from build123d import *

# Parameters (mm, degrees)
SKETCH1_W           = 5
SKETCH1_H           = 159
BOSS_EXTRUDE1_DEPTH = 3
SKETCH3_W           = 23
SKETCH3_H           = 5
BOSS_EXTRUDE2_DEPTH = 3
SKETCH5_R           = 1
CUT_EXTRUDE4_DEPTH  = 3


with BuildPart() as part:
    # Sketch1 → Boss-Extrude1 (new body)
    with BuildSketch(Plane(origin=(0, 0, 0), x_dir=(1, 0, 0), z_dir=(0, 1, 0))):
        with Locations((2.5, 79.5)):
            Rectangle(SKETCH1_W, SKETCH1_H)
    extrude(amount=BOSS_EXTRUDE1_DEPTH)

    # Sketch3 → Boss-Extrude2 (add)
    with BuildSketch(Plane(origin=(0, 0, 0), x_dir=(1, 0, 0), z_dir=(0, 1, 0))):
        with Locations((2.5, 12.5)):
            Rectangle(SKETCH3_W, SKETCH3_H)
        with Locations((2.5, 146.5)):
            Rectangle(SKETCH3_W, SKETCH3_H)
    extrude(amount=BOSS_EXTRUDE2_DEPTH)

    # Sketch5 → Cut-Extrude4 (cut)
    with BuildSketch(Plane(origin=(0, 0, 0), x_dir=(1, 0, 0), z_dir=(0, 1, 0))):
        with Locations((2.5, 12.5)):
            Circle(SKETCH5_R)
        with Locations((2.5, 146.5)):
            Circle(SKETCH5_R)
    extrude(amount=CUT_EXTRUDE4_DEPTH, mode=Mode.SUBTRACT)


solid = part.part
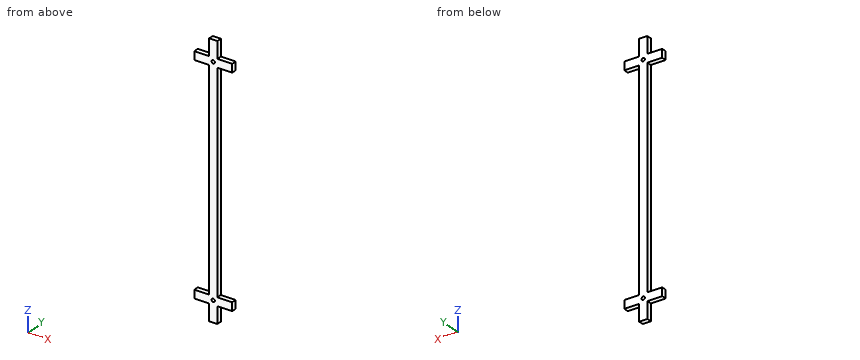
Can you work these out from the model? Positions are in its coordinate system, mm. Round coordinates to 2 decimals unless told otherwise and drop trailing zeros. Loops run counter-clockwise (first coordinate to the right, second up) from the corner with the lowest first, then second, coordinate; pieces in that order, holes last. Notation, with made-up numbers: (7, 2) - (49, 2) arc R15 cw to (49, 7) - close; hole circle Ø3 at (43.25, 2.25). An arc over 180 degrees is marked (long way). Write item = value, one per line. Start each with the question number.
(1) If we section it at A-A (y = 0.7): Please give me the cut outline in (x, z), and give its area (3 significant figures).
(2) If we section it at B-B (x = -2.75): Please give me the cut outline in (y, z), and give its area (3 significant figures).
(3) If we section it at C-C (z = -120.5): Please give me the cut outline in (x, y), and give its area (3 significant figures).
(4) If I drill on probe 1 along Z at (x, y) = (2.5, 1.5); probe 2 along Z at (x, y) = (-2.5, 0.9); probe 3 along X at (y, z) = (2.3, -146.5), over which ranges is the centre line in solid material (lowest first)? Write a range as [from, to].
(5) For P1, Ø0.9, axis at x = -2.5, y = 1, coming from the -Z side; P2, Ø1, axis at x = -2.5, y = 1.5, coming from the +Z side; P3, Ø1.5, axis at y = 1.5, z = -48, coming from the -X side, each with a flat end and sliding along its axis, tell me the tip position at first contact or that it passes through.
Ans:
q1.outline = (-9, -149) - (0, -149) - (0, -159) - (5, -159) - (5, -149) - (14, -149) - (14, -144) - (5, -144) - (5, -15) - (14, -15) - (14, -10) - (5, -10) - (5, 0) - (0, 0) - (0, -10) - (-9, -10) - (-9, -15) - (0, -15) - (0, -144) - (-9, -144) - close; hole circle Ø2 at (2.5, -146.5); hole circle Ø2 at (2.5, -12.5)
q1.area = 969 mm²
q2.outline = (0, -149) - (3, -149) - (3, -144) - (0, -144) - close; (0, -15) - (3, -15) - (3, -10) - (0, -10) - close
q2.area = 30.0 mm²
q3.outline = (0, 0) - (5, 0) - (5, 3) - (0, 3) - close
q3.area = 15.0 mm²
q4.probe_1 = [-159, -147.5], [-145.5, -13.5], [-11.5, 0]
q4.probe_2 = [-149, -144], [-15, -10]
q4.probe_3 = [-9, 1.5], [3.5, 14]
q5.P1 = -149
q5.P2 = -10
q5.P3 = 0
